Answer from the drawing. Dimensions are ordinates in mm from the lowest x, y and z of the part. A direction names the side the tool comes from. Coordinates: 2 decimals unless noted, no trailing zeros. Order: outer loops, then holes, each group sorted by start corner. A loop starts at its lowest first (then second) coordinate and runs counter-clockwise, first axis right, second up.
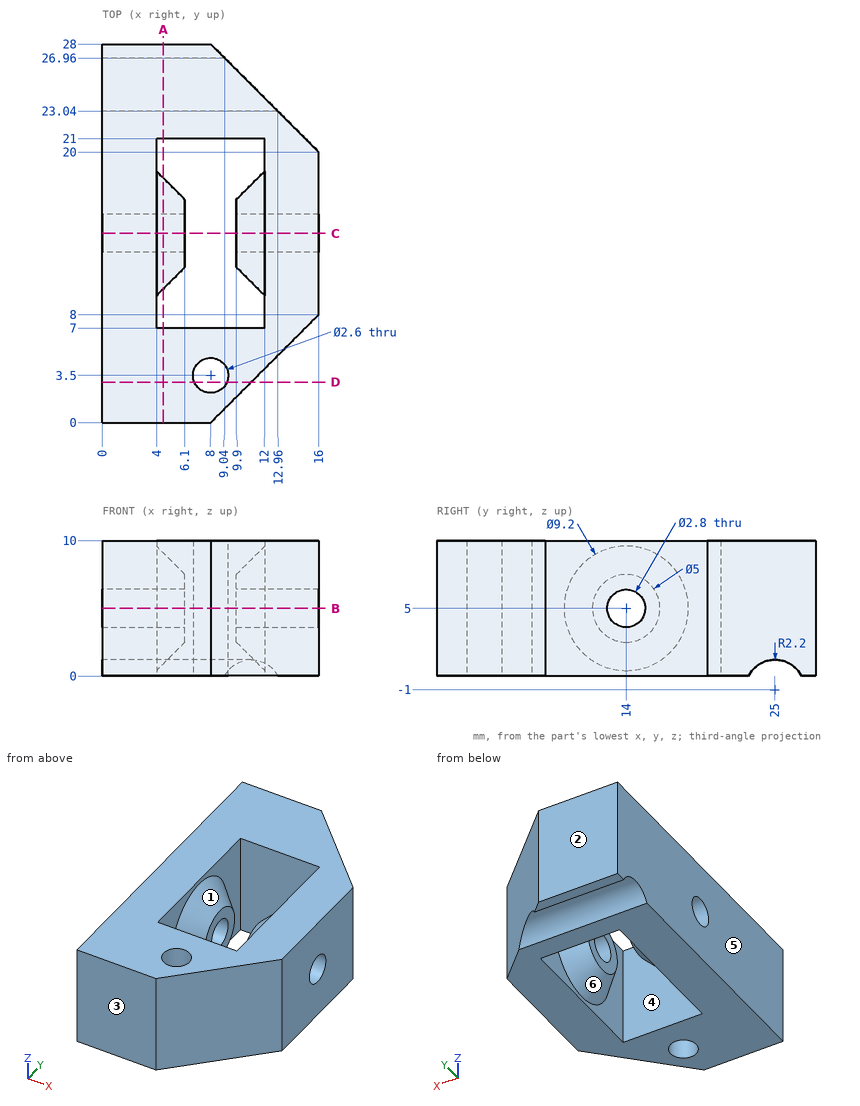
1) Section C-C (y = 14) is taken. Give the vertices of the cut face in (x, z).
2) Determine the mould class of the marked faces 1, 2 and 3 for opening direction Y: released by +Y, released by -Y, zero draft, split by the parting line, or undercut.
3) This flat-tipped pin is pushed along its axis until it touches: P1, Ø2, axis at y = 14, z = 5, coming from the +X side. Where does it stop, or does it pass through?
4) A tool of negligible diameter and unlimited length cuts with its end or side. For the marked faces 4, 5 and 6, from which of +Z, -Z, +X, -X, +Y, -Y can it reach the whole face along a straight path? Write none if from no direction.
5) Section B-B (z = 5) is taken. Give the vertices of the cut face in (x, y), then the cut area to 3 significant figures.
6) Consider L1, parallel to Y at x = 3.5, z = 5; L2, parallel to Z at x = 14.25, y = 14; L3, parallel to Y at x = 5, z = 5.75. Determine where each line is inside the solid, lowest interval first.
7) Section D-D (y = 3) is taken. Give the vertices of the cut face in (x, z).
8) Section A-A (x = 4.5) is taken. Give the vertices of the cut face in (y, z).
Filled sheet:
1. outline: (0, 0) - (4, 0) - (4, 0.4) - (6.1, 2.5) - (6.1, 3.6) - (0, 3.6) - close; (0, 6.4) - (6.1, 6.4) - (6.1, 7.5) - (4, 9.6) - (4, 10) - (0, 10) - close; (9.9, 2.5) - (12, 0.4) - (12, 0) - (16, 0) - (16, 3.6) - (9.9, 3.6) - close; (9.9, 6.4) - (16, 6.4) - (16, 10) - (12, 10) - (12, 9.6) - (9.9, 7.5) - close
2. face 1: undercut
2. face 2: released by +Y
2. face 3: released by -Y
3. P1: passes through
4. face 4: +Z, -Z
4. face 5: +Z, -Z, -X, +Y, -Y
4. face 6: none
5. outline: (0, 0) - (8, 0) - (16, 8) - (16, 12.6) - (9.9, 12.6) - (9.9, 11.5) - (12, 9.4) - (12, 7) - (4, 7) - (4, 9.4) - (6.1, 11.5) - (6.1, 12.6) - (0, 12.6) - close; (0, 15.4) - (6.1, 15.4) - (6.1, 16.5) - (4, 18.6) - (4, 21) - (12, 21) - (12, 18.6) - (9.9, 16.5) - (9.9, 15.4) - (16, 15.4) - (16, 20) - (8, 28) - (0, 28) - close; hole circle Ø2.6 at (8, 3.5)
5. area: 262 mm2
6. L1: y = 0 to 12.6, 15.4 to 28
6. L2: z = 0 to 3.6, 6.4 to 10
6. L3: y = 0 to 7, 10.48 to 12.82, 15.18 to 17.52, 21 to 28
7. outline: (0, 0) - (6.8, 0) - (6.8, 10) - (0, 10) - close; (9.2, 0) - (11, 0) - (11, 10) - (9.2, 10) - close
8. outline: (0, 0) - (7, 0) - (7, 10) - (0, 10) - close; circle Ø8.2 at (14, 5); (21, 0) - (23.04, 0) arc R2.2 cw to (26.96, 0) - (28, 0) - (28, 10) - (21, 10) - close; hole circle Ø2.8 at (14, 5)
